Input: part model. Units: mm. Frame: model coordinates. A direction names the side the tool comes from. Round coordinates to 2 decimals unless told otherwise and drop trailing zeros. Loops run counter-clockwise (first coordinate to the right, second up) from the corner with the lowest first, then second, coordinate; pieces in that order, holes last. Notation, with made-up numbers: M 40.5,6.5 L 90.5,6.5 A19 cw 90.5,38.5 Z; hole C -11.5,57.25 d3. An arc over 180 degrees is marked long. Use one line per item in the form item = value. Start each with the question number.
Q1. Section query D-D, the plane y = 26. Output: boundary loops of the cut face in (x, z), and give its area (3 significant figures).
Q2. Mould query, pull axis X, two halves, no side actions, for faces 3 (the flat face through (4, 60, 10)), 4 (the cylindrical face through (7.466, 1.479, 6.237)), 5 (the cylindrical face through (48.01, 29.58, -5.11)). Classes: pulls with the +X half, pulls with the -X half, needs draft (parallel to the pull), parting line crosses it, or undercut.
Q3. Ray query, line 1 along X through (y, z) = (51.5, 4.25); line 2 along X through (y, z) = (54, 2.5); line 3 along Z through (x, y) = (-11, 23.5). Return the intervals inside material, ascending.
Q4. Section query B-B, the plane y = 8.5. Output: boundary loops of the cut face in (x, z).
Q5. First-contact query: P1, Ø2, axis at y = 34.5, z = 10.5, coming from the -X side; P2, Ø3, axis at y = 31, z = 1, coming from the +X side; P3, Ø5, axis at y = 15, z = 4, coming from the +X side; P4, Ø11.5, axis at x = -6, z = -5.5, coming from the +Y side. Flat tips, straight axial feed; report the tip coordinate or a pass-through.
Q6. Access query for faces 1 (the cylindrical face through (4.065, 1.479, 0.534)), 2 (the flat face through (0, 33.5, 11)). Directions: +Z, -Z, +X, -X, +Y, -Y. A direction counts if a zero-diameter tool reaches every point of the face in a straight line with its end or side. Return the directions, or none.
Q7. Section query A-A, the plane y = 34.5. Output: boundary loops of the cut face in (x, z).
Q8. Section query C-C, the plane x = 3. Output: boundary loops of the cut face in (y, z), and give its area (3 significant figures).
```python
from build123d import *

# Parameters (mm, degrees)
BOSS_EXTRUDE1_DEPTH = 60
SKETCH2_R           = 9.5
CUT_EXTRUDE1_DEPTH  = 60
CUT_EXTRUDE2_DEPTH  = 60
BOSS_EXTRUDE3_DEPTH = 3
SKETCH5_R           = 4.1
CUT_EXTRUDE3_DEPTH  = 3
SKETCH6_R           = 1.5
CUT_EXTRUDE4_DEPTH  = 3
SKETCH8_R           = 1.5
SKETCH8_W           = 10
SKETCH8_H           = 3
CUT_EXTRUDE5_DEPTH  = 3
FILLET1_R           = 1


with BuildPart() as part:
    # Sketch1 → Boss-Extrude1 (new body)
    with BuildSketch(Plane(origin=(0, 0, 0), x_dir=(1, 0, 0), z_dir=(0, 1, 0))):
        with BuildLine():
            Line((-40, 11.5), (40, 11.5))
            ThreePointArc((40, 11.5), (51.5, 0), (40, -11.5))
            Line((40, -11.5), (-40, -11.5))
            ThreePointArc((-40, -11.5), (-51.5, 0), (-40, 11.5))
        make_face()
    extrude(amount=BOSS_EXTRUDE1_DEPTH)

    # Sketch2 → Cut-Extrude1 (cut)
    with BuildSketch(Plane.XZ):
        with Locations(Location((-40, 0, 0), (0, 0, 270))):
            Circle(SKETCH2_R)
        with Locations(Location((40, 0, 0), (0, 0, 270))):
            Circle(SKETCH2_R)
    extrude(amount=-CUT_EXTRUDE1_DEPTH, mode=Mode.SUBTRACT)

    # Sketch3 → Cut-Extrude2 (cut)
    with BuildSketch(Plane.XZ):
        with BuildLine():
            Line((33.519259302, 9.5), (-33.519259302, 9.5))
            ThreePointArc((-33.519259302, 9.5), (-29.831949104, 5.372219372), (-28.5, 0))
            ThreePointArc((-28.5, 0), (-31.868272016, -8.131727984), (-40, -11.5))
            Line((-40, -11.5), (40, -11.5))
            ThreePointArc((40, -11.5), (29.011369512, -3.391164992), (33.519259302, 9.5))
        make_face()
    extrude(amount=-CUT_EXTRUDE2_DEPTH, mode=Mode.SUBTRACT)

    # Sketch4 → Boss-Extrude3 (add)
    with BuildSketch(Plane.XZ):
        with BuildLine():
            Line((-33.519259302, 9.5), (33.519259302, 9.5))
            ThreePointArc((33.519259302, 9.5), (21.099049386, 5.75486124), (12.819526766, -4.231989308))
            ThreePointArc((12.819526766, -4.231989308), (0, -13.5), (-12.819526766, -4.231989308))
            ThreePointArc((-12.819526766, -4.231989308), (-21.099049386, 5.75486124), (-33.519259302, 9.5))
        make_face()
    extrude(amount=-BOSS_EXTRUDE3_DEPTH)

    # Sketch5 → Cut-Extrude3 (cut)
    with BuildSketch(Plane.XZ):
        with Locations(Location((0, 0, 0), (0, 0, 270))):
            Circle(SKETCH5_R)
    extrude(amount=-CUT_EXTRUDE3_DEPTH, mode=Mode.SUBTRACT)

    # Sketch6 → Cut-Extrude4 (cut)
    with BuildSketch(Plane.XZ):
        with Locations(Location((5.979202711, -6.041451394, 0), (0, 0, 270))):
            Circle(SKETCH6_R)
        with Locations(Location((-6.020797289, -6, 0), (0, 0, 270))):
            Circle(SKETCH6_R)
        with Locations(Location((-6.020797289, 6, 0), (0, 0, 270))):
            Circle(SKETCH6_R)
        with Locations(Location((5.979202711, 6.041451394, 0), (0, 0, 270))):
            Circle(SKETCH6_R)
    extrude(amount=-CUT_EXTRUDE4_DEPTH, mode=Mode.SUBTRACT)

    # Sketch8 → Cut-Extrude5 (cut)
    with BuildSketch(Plane.XY.offset(11.5)):
        with Locations((3, 26)):
            Circle(SKETCH8_R)
        with Locations((0, 35)):
            Rectangle(SKETCH8_W, SKETCH8_H)
    extrude(amount=-CUT_EXTRUDE5_DEPTH, mode=Mode.SUBTRACT)

    # Fillet1
    fillet1_edges = [part.edges().sort_by_distance(p)[0] for p in [
        (-40, 0, 9.5),
    ]]
    fillet(fillet1_edges, radius=FILLET1_R)


solid = part.part
```
Results found:
q1.outline = M -40,11.5 A11.5 ccw long -33.52,9.5 L 1.5,9.5 L 1.5,11.5 Z; M 4.5,9.5 L 33.52,9.5 A11.5 ccw long 40,11.5 L 4.5,11.5 Z; hole C -40,0 d19; hole C 40,0 d19
q1.area = 400 mm²
q2.face_3 = needs draft
q2.face_4 = undercut
q2.face_5 = undercut
q3.line_1 = -50.69 to -48.5, -31.5 to -29.31, 29.31 to 31.5, 48.5 to 50.69
q3.line_2 = -51.22 to -49.17, -30.83 to -28.78, 28.78 to 30.83, 49.17 to 51.22
q3.line_3 = 9.5 to 11.5
q4.outline = M -40,11.5 A11.5 ccw long -33.52,9.5 L 33.52,9.5 A11.5 ccw long 40,11.5 Z; hole C -40,0 d19; hole C 40,0 d19
q5.P1 = -46.48
q5.P2 = 51.5
q5.P3 = 51.4
q5.P4 = 3
q6.face_1 = +Y, -Y
q6.face_2 = +Z, -Z
q7.outline = M -40,11.5 A11.5 ccw long -33.52,9.5 L -5,9.5 L -5,11.5 Z; M 5,9.5 L 33.52,9.5 A11.5 ccw long 40,11.5 L 5,11.5 Z; hole C -40,0 d19; hole C 40,0 d19
q8.outline = M 0,-13.16 L 3,-13.16 L 3,-2.79 L 0,-2.79 Z; M 0,2.79 L 3,2.79 L 3,9.5 L 24.5,9.5 L 24.5,11.5 L 0,11.5 Z; M 27.5,9.5 L 33.5,9.5 L 33.5,11.5 L 27.5,11.5 Z; M 36.5,9.5 L 60,9.5 L 60,11.5 L 36.5,11.5 Z
q8.area = 159 mm²
